Input: part model. Units: mm. Frame: model coordinates. A direction names the side the tool comes from. Round coordinates to 2 decimals unless told otherwise and drop trailing zeros. Loops run counter-clockwise (first coordinate to the right, second up) from the corner with the lowest first, then second, coordinate; pieces in that order, holes last. Notation, with made-up numbers: (-20.75, -18) -> (1.25, -18) arc R27 cw to (1.25, 6) -> close; hole circle Ø5 at (29, -19). An arc over 180 degrees is marked (long way). Answer as a JSON object with one key per item and string values.
```python
from build123d import *

# Parameters (mm, degrees)
BOSS_EXTRUDE1_DEPTH = 48
SKETCH2_R           = 2
CUT_EXTRUDE1_DEPTH  = 48
SKETCH3_R           = 11
BOSS_EXTRUDE2_DEPTH = 2
SKETCH4_R           = 2.5
BOSS_EXTRUDE3_DEPTH = 22
CUT_EXTRUDE2_START  = -15
CUT_EXTRUDE2_DEPTH  = 15
SKETCH6_R           = 1.5875
CUT_EXTRUDE5_DEPTH  = 79.623819546
BOSS_EXTRUDE4_START = 10
SKETCH7_R           = 2.5
BOSS_EXTRUDE4_DEPTH = 10
SKETCH8_R           = 0.75
CUT_EXTRUDE6_DEPTH  = 10


with BuildPart() as part:
    # Sketch1 → Boss-Extrude1 (new body)
    with BuildSketch(Plane(origin=(0, 0, 0), x_dir=(1, 0, 0), z_dir=(0, 1, 0))):
        Polygon((16.807359313, -21.05), (21.05, -16.807359313), (21.05, 16.807359313), (16.807359313, 21.05), (-16.807359313, 21.05), (-21.05, 16.807359313), (-21.05, -16.807359313), (-16.807359313, -21.05), align=None)
    extrude(amount=BOSS_EXTRUDE1_DEPTH)

    # Sketch2 → Cut-Extrude1 (cut)
    with BuildSketch(Plane(origin=(0, 48, 0), x_dir=(1, 0, 0), z_dir=(0, 1, 0))):
        with Locations(Location((-15.5, 15.5, 0), (0, 0, 270))):
            Circle(SKETCH2_R)
        with Locations(Location((15.5, 15.5, 0), (0, 0, 90))):
            Circle(SKETCH2_R)
        with Locations(Location((15.5, -15.5, 0), (0, 0, 270))):
            Circle(SKETCH2_R)
        with Locations(Location((-15.5, -15.5, 0), (0, 0, 90))):
            Circle(SKETCH2_R)
    extrude(amount=-CUT_EXTRUDE1_DEPTH, mode=Mode.SUBTRACT)

    # Sketch3 → Boss-Extrude2 (add)
    with BuildSketch(Plane(origin=(0, 48, 0), x_dir=(1, 0, 0), z_dir=(0, 1, 0))):
        with Locations(Location((0, 0, 0), (0, 0, 90))):
            Circle(SKETCH3_R)
    extrude(amount=BOSS_EXTRUDE2_DEPTH)

    # Sketch4 → Boss-Extrude3 (add)
    with BuildSketch(Plane(origin=(0, 50, 0), x_dir=(1, 0, 0), z_dir=(0, 1, 0))):
        with Locations(Location((0, 0, 0), (0, 0, 270))):
            Circle(SKETCH4_R)
    extrude(amount=BOSS_EXTRUDE3_DEPTH)

    # Sketch5 → Cut-Extrude2 (cut)
    with BuildSketch(Plane(origin=(0, 72, 0), x_dir=(1, 0, 0), z_dir=(0, 1, 0)).offset(CUT_EXTRUDE2_START)):
        with BuildLine():
            Line((-1.5, 2), (1.5, 2))
            ThreePointArc((1.5, 2), (0, 2.5), (-1.5, 2))
        make_face()
    extrude(amount=CUT_EXTRUDE2_DEPTH, mode=Mode.SUBTRACT)

    # Sketch6 → Cut-Extrude5 (cut, through all)
    with BuildSketch(Plane(origin=(0, 0, -2.5), x_dir=(-1, 0, 0), z_dir=(0, 0, -1))):
        with Locations((0, 54.5875)):
            Circle(SKETCH6_R)
    extrude(amount=-CUT_EXTRUDE5_DEPTH, mode=Mode.SUBTRACT)

    # Sketch7 → Boss-Extrude4 (add)
    with BuildSketch(Plane.XZ.offset(BOSS_EXTRUDE4_START)):
        with Locations(Location((0, 0, 0), (0, 0, 233.130102354))):
            Circle(SKETCH7_R)
    extrude(amount=-BOSS_EXTRUDE4_DEPTH)

    # Sketch8 → Cut-Extrude6 (cut)
    with BuildSketch(Plane.XZ.offset(10)):
        with Locations(Location((0, 0, 0), (0, 0, 270))):
            Circle(SKETCH8_R)
    extrude(amount=-CUT_EXTRUDE6_DEPTH, mode=Mode.SUBTRACT)


solid = part.part
```
1) Section A-A, the plane x = 15.5. Output: boundary loops of the cut face in (y, z).
Output:
{"outline": "(0, -21.05) -> (48, -21.05) -> (48, -17.5) -> (0, -17.5) -> close; (0, -13.5) -> (48, -13.5) -> (48, 13.5) -> (0, 13.5) -> close; (0, 17.5) -> (48, 17.5) -> (48, 21.05) -> (0, 21.05) -> close"}
2) Section C-C, the plane z = 15.5. Output: boundary loops of the cut face in (x, y), plus the area to 3 significant figures.
Output:
{"outline": "(-21.05, 0) -> (-17.5, 0) -> (-17.5, 48) -> (-21.05, 48) -> close; (-13.5, 0) -> (13.5, 0) -> (13.5, 48) -> (-13.5, 48) -> close; (17.5, 0) -> (21.05, 0) -> (21.05, 48) -> (17.5, 48) -> close", "area": "1,640 mm^2"}
3) Reachability of faces 1 (the face through (-13.517, 24.336, -15.76)), 2 (the face through (-2.467, -5.07, 0.408)), 3 (the face through (0, 64, -2)), 4 (the face through (10.74, 48.99, 2.38)) from +Z, -Z, +X, -X, +Y, -Y: full face, straight path, thin tool, end or side. Return the list, or none.
Output:
{"face 1": "+Y, -Y", "face 2": "-Y", "face 3": "-Z, +X, -X, +Y", "face 4": "+Y"}
4) Section D-D, the plane x = -8. Output: boundary loops of the cut face in (y, z), plus the area to 3 significant figures.
Output:
{"outline": "(0, -21.05) -> (48, -21.05) -> (48, -7.55) -> (50, -7.55) -> (50, 7.55) -> (48, 7.55) -> (48, 21.05) -> (0, 21.05) -> close", "area": "2,050 mm^2"}
5) Contact query for flat-ended pins moving along their axis: P1, Ø3, axis at x = 15.5, z = 15.5, coming from the -Y side; P2, Ø4.5, axis at x = -15.5, z = -15.5, coming from the -Y side; P3, Ø2.5, axis at x = 0, z = 0, coming from the -Y side; P4, Ø3.5, axis at x = 0.5, y = 64.5, coming from the -Z side. Output: stop coordinate, or through.
Output:
{"P1": "passes through", "P2": "stops at y = 0", "P3": "stops at y = -10", "P4": "stops at z = -2"}
6) Section B-B, the plane y = 23. Output: boundary loops of the cut face in (x, z), plus the area to 3 significant figures.
Output:
{"outline": "(-21.05, -16.81) -> (-16.81, -21.05) -> (16.81, -21.05) -> (21.05, -16.81) -> (21.05, 16.81) -> (16.81, 21.05) -> (-16.81, 21.05) -> (-21.05, 16.81) -> close; hole circle Ø4 at (-15.5, -15.5); hole circle Ø4 at (-15.5, 15.5); hole circle Ø4 at (15.5, -15.5); hole circle Ø4 at (15.5, 15.5)", "area": "1,690 mm^2"}
7) Ray query, probe 1 along X at (y, z) = (14, 15.5); probe 2 along X at (y, z) = (35, 15); probe 3 along Y at (x, z) = (15.5, -12.5). Return the intervals inside material, ascending.
Output:
{"probe 1": "x = -21.05 to -17.5, -13.5 to 13.5, 17.5 to 21.05", "probe 2": "x = -21.05 to -17.44, -13.56 to 13.56, 17.44 to 21.05", "probe 3": "y = 0 to 48"}
8) Draft query along X for faces 5 (the face through (-0.96, 60.85, 2.31)), 6 (the face through (-0.85, 55.93, -0.04)), 7 (the face through (0, -10, -1)). Return one class per face: +X half, -X half, draft (parallel to the pull), parting line (faces both ways), or undercut.
Output:
{"face 5": "parting line", "face 6": "undercut", "face 7": "draft"}
